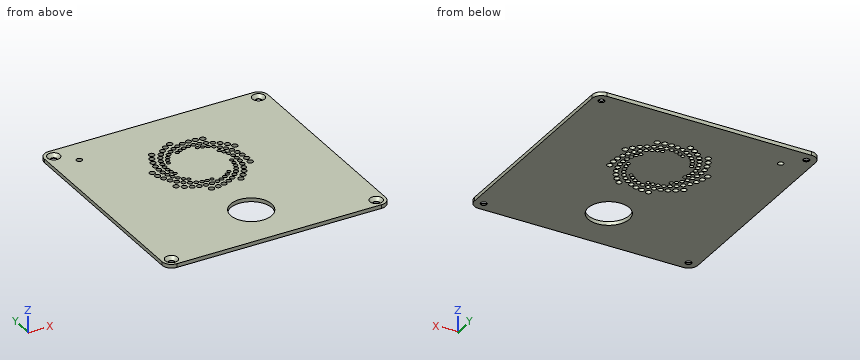
from build123d import *

# Parameters (mm, degrees)
F0_R           = 1.5
F0_R_2         = 1.4
F0_R_3         = 1.35
F0_R_4         = 1.45
F0_R_5         = 1.3
F0_R_6         = 1.05
F0_R_7         = 1.25
F0_R_8         = 1.2
F0_R_9         = 1
F0_R_10        = 11
F0_R_11        = 1.15
F0_R_12        = 1.1
F1_DEPTH       = 2
F3_D           = 3.3
F3_CSINK_D     = 6.72
F3_CSINK_ANGLE = 90


with BuildPart() as f1:
    # F0 (on Top) → F1 (new body)
    with BuildSketch(Plane.XY):
        with BuildLine():
            Line((-55, -60), (55, -60))
            ThreePointArc((55, -60), (58.5355339059, -58.5355339059), (60, -55))
            Line((60, -55), (60, 55))
            ThreePointArc((60, 55), (58.5355339059, 58.5355339059), (55, 60))
            Line((55, 60), (-55, 60))
            ThreePointArc((-55, 60), (-58.5355339059, 58.5355339059), (-60, 55))
            Line((-60, 55), (-60, -55))
            ThreePointArc((-60, -55), (-58.5355339059, -58.5355339059), (-55, -60))
        make_face()
        with Locations((-6.2195005757, -7.5245201893)):
            Circle(F0_R, mode=Mode.SUBTRACT)
        with Locations((-13.2095659082, -1.6022741634)):
            Circle(F0_R_2, mode=Mode.SUBTRACT)
        with Locations((-9.9718863075, -2.7407789908)):
            Circle(F0_R_3, mode=Mode.SUBTRACT)
        with Locations((-2.4208439444, -7.2535090453)):
            Circle(F0_R_4, mode=Mode.SUBTRACT)
        with Locations((-6.744894099, -3.34734333)):
            Circle(F0_R_5, mode=Mode.SUBTRACT)
        with Locations((-4.2086559278, -0.0616157499)):
            Circle(F0_R_6, mode=Mode.SUBTRACT)
        with Locations((-3.5667660577, -3.4381477467)):
            Circle(F0_R_7, mode=Mode.SUBTRACT)
        with Locations((-0.4794412689, -3.0295308984)):
            Circle(F0_R_8, mode=Mode.SUBTRACT)
        with Locations((-1.6394864233, -0.0045228822)):
            Circle(F0_R_9, mode=Mode.SUBTRACT)
        with Locations((0, -33.8560082018)):
            Circle(F0_R_10, mode=Mode.SUBTRACT)
        with Locations((1.0897714947, -6.5685119785)):
            Circle(F0_R_2, mode=Mode.SUBTRACT)
        with Locations((4.320428574, -5.2589490383)):
            Circle(F0_R_3, mode=Mode.SUBTRACT)
        with Locations((2.2446686472, -2.2122976675)):
            Circle(F0_R_11, mode=Mode.SUBTRACT)
        with Locations((7.1572727593, -3.5527772575)):
            Circle(F0_R_5, mode=Mode.SUBTRACT)
        with Locations((4.7417693841, -1.0318500295)):
            Circle(F0_R_12, mode=Mode.SUBTRACT)
        with Locations((10.2772820811, -6.3879620589)):
            Circle(F0_R, mode=Mode.SUBTRACT)
        with Locations((12.9488032381, -3.785707087)):
            Circle(F0_R_4, mode=Mode.SUBTRACT)
        with Locations((9.6169902081, -1.4934791557)):
            Circle(F0_R_7, mode=Mode.SUBTRACT)
        with Locations((15.0894230301, -0.8744641978)):
            Circle(F0_R_2, mode=Mode.SUBTRACT)
        with Locations((-19.4530965691, 2.4914951923)):
            Circle(F0_R, mode=Mode.SUBTRACT)
        with Locations((-16.4204941993, 0.1530332652)):
            Circle(F0_R_4, mode=Mode.SUBTRACT)
        with Locations((-17.0878687804, 6.0222702727)):
            Circle(F0_R_5, mode=Mode.SUBTRACT)
        with Locations((-19.1888803547, 8.5759251074)):
            Circle(F0_R_3, mode=Mode.SUBTRACT)
        with Locations((-16.3817511802, 11.1066447266)):
            Circle(F0_R_11, mode=Mode.SUBTRACT)
        with Locations((-20.8378577535, 11.6811562025)):
            Circle(F0_R_2, mode=Mode.SUBTRACT)
        with Locations((-17.6128627663, 13.7632745013)):
            Circle(F0_R_8, mode=Mode.SUBTRACT)
        with Locations((-12.1751217102, 2.1627622468)):
            Circle(F0_R_8, mode=Mode.SUBTRACT)
        with Locations((-9.5412278478, 0.9805144786)):
            Circle(F0_R_11, mode=Mode.SUBTRACT)
        with Locations((-14.7391617229, 3.8671595671)):
            Circle(F0_R_7, mode=Mode.SUBTRACT)
        with Locations((-13.0009319564, 6.7895073139)):
            Circle(F0_R_6, mode=Mode.SUBTRACT)
        with Locations((-11.0597781767, 5.2480040745)):
            Circle(F0_R_9, mode=Mode.SUBTRACT)
        with Locations((-6.8349194643, 0.2238475413)):
            Circle(F0_R_12, mode=Mode.SUBTRACT)
        with Locations((-14.8278962751, 8.7877511673)):
            Circle(F0_R_12, mode=Mode.SUBTRACT)
        with Locations((-13.9144141157, 13.0126103454)):
            Circle(F0_R_9, mode=Mode.SUBTRACT)
        with Locations((-22.9111540993, 18.7842817672)):
            Circle(F0_R, mode=Mode.SUBTRACT)
        with Locations((-22.1386555513, 15.0655554303)):
            Circle(F0_R_4, mode=Mode.SUBTRACT)
        with Locations((-18.4427140211, 16.7031753503)):
            Circle(F0_R_7, mode=Mode.SUBTRACT)
        with Locations((-15.2037231182, 17.8747428276)):
            Circle(F0_R_12, mode=Mode.SUBTRACT)
        with Locations((-18.7601869856, 19.8778332838)):
            Circle(F0_R_5, mode=Mode.SUBTRACT)
        with Locations((-15.2653934364, 20.5665165254)):
            Circle(F0_R_11, mode=Mode.SUBTRACT)
        with Locations((-18.6333035981, 23.230218298)):
            Circle(F0_R_3, mode=Mode.SUBTRACT)
        with Locations((-17.9479293456, 26.7000375011)):
            Circle(F0_R_2, mode=Mode.SUBTRACT)
        with Locations((-14.7137114709, 15.2963185378)):
            Circle(F0_R_6, mode=Mode.SUBTRACT)
        with Locations((-14.9147607317, 23.3061620661)):
            Circle(F0_R_8, mode=Mode.SUBTRACT)
        with Locations((-11.7448925902, 23.1180181422)):
            Circle(F0_R_9, mode=Mode.SUBTRACT)
        with Locations((-14.0882221912, 26.1341565915)):
            Circle(F0_R_7, mode=Mode.SUBTRACT)
        with Locations((-10.8314094995, 25.4017254033)):
            Circle(F0_R_6, mode=Mode.SUBTRACT)
        with Locations((-12.71951142, 28.9193587073)):
            Circle(F0_R_5, mode=Mode.SUBTRACT)
        with Locations((-9.5481708576, 27.6238368519)):
            Circle(F0_R_12, mode=Mode.SUBTRACT)
        with Locations((-7.8182857414, 29.7311963209)):
            Circle(F0_R_11, mode=Mode.SUBTRACT)
        with Locations((-3.4150964511, 29.3566630848)):
            Circle(F0_R_9, mode=Mode.SUBTRACT)
        with Locations((-46.3356375694, 46.1809411645)):
            Circle(F0_R, mode=Mode.SUBTRACT)
        with Locations((-16.6427524691, 30.0739695944)):
            Circle(F0_R_4, mode=Mode.SUBTRACT)
        with Locations((-14.7720783879, 33.4214912423)):
            Circle(F0_R, mode=Mode.SUBTRACT)
        with Locations((-10.9200630267, 31.5629942038)):
            Circle(F0_R_3, mode=Mode.SUBTRACT)
        with Locations((-8.6085241218, 34.0252527662)):
            Circle(F0_R_2, mode=Mode.SUBTRACT)
        with Locations((-5.6933987816, 31.6130080887)):
            Circle(F0_R_8, mode=Mode.SUBTRACT)
        with Locations((-1.2505264185, 30.511100746)):
            Circle(F0_R_6, mode=Mode.SUBTRACT)
        with Locations((-3.2400753279, 33.194542832)):
            Circle(F0_R_7, mode=Mode.SUBTRACT)
        with Locations((-5.8125317027, 36.1782768436)):
            Circle(F0_R_4, mode=Mode.SUBTRACT)
        with Locations((-0.3653573385, 34.4533966549)):
            Circle(F0_R_5, mode=Mode.SUBTRACT)
        with Locations((-2.5428621029, 37.9275539585)):
            Circle(F0_R, mode=Mode.SUBTRACT)
        with Locations((6.9210576894, 0.5118121321)):
            Circle(F0_R_6, mode=Mode.SUBTRACT)
        with Locations((8.7371306563, 2.1916801038)):
            Circle(F0_R_9, mode=Mode.SUBTRACT)
        with Locations((11.6190860118, 0.680224532)):
            Circle(F0_R_8, mode=Mode.SUBTRACT)
        with Locations((13.1635587732, 3.0827383439)):
            Circle(F0_R_11, mode=Mode.SUBTRACT)
        with Locations((14.2504103551, 5.5996579744)):
            Circle(F0_R_12, mode=Mode.SUBTRACT)
        with Locations((14.8796407575, 8.173780951)):
            Circle(F0_R_6, mode=Mode.SUBTRACT)
        with Locations((16.673070013, 2.1594428385)):
            Circle(F0_R_3, mode=Mode.SUBTRACT)
        with Locations((17.7397770877, 5.3136446208)):
            Circle(F0_R_5, mode=Mode.SUBTRACT)
        with Locations((21.916254058, 5.254852555)):
            Circle(F0_R, mode=Mode.SUBTRACT)
        with Locations((18.2546028937, 8.4025920064)):
            Circle(F0_R_7, mode=Mode.SUBTRACT)
        with Locations((15.1656545768, 10.7479039275)):
            Circle(F0_R_9, mode=Mode.SUBTRACT)
        with Locations((22.1859557624, 8.9767276936)):
            Circle(F0_R_4, mode=Mode.SUBTRACT)
        with Locations((18.2546028937, 11.3771333986)):
            Circle(F0_R_8, mode=Mode.SUBTRACT)
        with Locations((17.8541826154, 14.1800669648)):
            Circle(F0_R_11, mode=Mode.SUBTRACT)
        with Locations((21.8965919758, 12.5258136236)):
            Circle(F0_R_2, mode=Mode.SUBTRACT)
        with Locations((14.422019578, 21.2160022624)):
            Circle(F0_R_9, mode=Mode.SUBTRACT)
        with Locations((6.9856644678, 28.5951541432)):
            Circle(F0_R_9, mode=Mode.SUBTRACT)
        with Locations((14.1360048274, 25.6206122853)):
            Circle(F0_R_11, mode=Mode.SUBTRACT)
        with Locations((9.3881791527, 28.0231265046)):
            Circle(F0_R_6, mode=Mode.SUBTRACT)
        with Locations((11.790693372, 27.0506804504)):
            Circle(F0_R_12, mode=Mode.SUBTRACT)
        with Locations((16.9961420889, 16.8685959347)):
            Circle(F0_R_12, mode=Mode.SUBTRACT)
        with Locations((21.1318308557, 15.8720388704)):
            Circle(F0_R_3, mode=Mode.SUBTRACT)
        with Locations((15.8520868118, 19.2139064588)):
            Circle(F0_R_6, mode=Mode.SUBTRACT)
        with Locations((18.1973991985, 21.502017013)):
            Circle(F0_R_7, mode=Mode.SUBTRACT)
        with Locations((19.856278419, 18.8706917383)):
            Circle(F0_R_5, mode=Mode.SUBTRACT)
        with Locations((23.0489993538, 21.5448019721)):
            Circle(F0_R, mode=Mode.SUBTRACT)
        with Locations((16.3097089226, 23.7901257046)):
            Circle(F0_R_8, mode=Mode.SUBTRACT)
        with Locations((20.8374491031, 24.5115132698)):
            Circle(F0_R_4, mode=Mode.SUBTRACT)
        with Locations((18.3107188041, 27.003996975)):
            Circle(F0_R_2, mode=Mode.SUBTRACT)
        with Locations((15.565852269, 28.9864027568)):
            Circle(F0_R_3, mode=Mode.SUBTRACT)
        with Locations((1.2507550837, 31.3288280435)):
            Circle(F0_R_12, mode=Mode.SUBTRACT)
        with Locations((3.8963412936, 31.7617421665)):
            Circle(F0_R_11, mode=Mode.SUBTRACT)
        with Locations((6.7343335668, 31.8098431148)):
            Circle(F0_R_8, mode=Mode.SUBTRACT)
        with Locations((2.7717143367, 35.2802173861)):
            Circle(F0_R_3, mode=Mode.SUBTRACT)
        with Locations((6.1476380634, 35.5577924915)):
            Circle(F0_R_2, mode=Mode.SUBTRACT)
        with Locations((9.6685295994, 31.3769289919)):
            Circle(F0_R_7, mode=Mode.SUBTRACT)
        with Locations((12.6508265803, 30.4148969867)):
            Circle(F0_R_5, mode=Mode.SUBTRACT)
        with Locations((9.6943719382, 35.3388571807)):
            Circle(F0_R_4, mode=Mode.SUBTRACT)
        with Locations((13.2880402216, 34.5373386212)):
            Circle(F0_R, mode=Mode.SUBTRACT)
    extrude(amount=F1_DEPTH)

    # F3 (through all)
    with Locations(Plane.XY.offset(2)):
        with Locations((-55, 55), (55, 55), (55, -55), (-55, -55)):
            CounterSinkHole(F3_D / 2, F3_CSINK_D / 2, counter_sink_angle=F3_CSINK_ANGLE)


solid = f1.part
Geometry: final body of the model. Coordinates: model frame, mm. Coordinates: 2 decimals unless noted, no trailing zeros. Write each loop counter-clockwise with the first axis right and the second up, starting at its lowest first coordinate (ties: lowest second). Pieces come first, ordered by that corner, then holes. Notation, with made-up numbers: (87, 61) - (127, 61) arc R32 ccw to (127, 91) - close; hole circle Ø3 at (43.5, -6.75). An arc over 180 degrees is marked (long way). Return JSON: item names as keys, results as strings.
Item 1: Pin query (flat end, axial travel): pin 1 Ø5.5 at (x, y) = (55, 55) entering from +Z. Return the tip coordinate at first contact, or that it passes through.
Completed:
{"pin 1": "stops at z = 1.39"}
Item 2: Line query: L1, parallel to X at y = 55, z = 0.1; L2, parallel to X at y = -34, z = 1.05; L3, parallel to X at y = -7, z = 1.4. Output: solid intervals per line, ascending.
Completed:
{"L1": "x = -60 to -56.65, -53.35 to 53.35, 56.65 to 60", "L2": "x = -60 to -11, 11 to 60", "L3": "x = -60 to -7.62, -4.81 to -3.85, -0.99 to -0.24, 2.42 to 8.91, 11.65 to 60"}
Item 3: Section query B-B (z = 0.8). Count the separate pieces of the cut face and the enclosed holes in it, and give its area (3 significant figures).
Completed:
{"separate pieces": "1", "enclosed holes": "105", "area": "13,400 mm2"}
Item 4: Section query A-A (y = -28.5). Output: boundary loops of the cut face in (x, z).
Completed:
{"outline": "(-60, 0) - (-9.61, 0) - (-9.61, 2) - (-60, 2) - close; (9.61, 0) - (60, 0) - (60, 2) - (9.61, 2) - close"}
